```python
from build123d import *

# Parameters (mm, degrees)
SKETCH1_W           = 79
SKETCH1_H           = 46
SKETCH1_W_2         = 10
SKETCH1_H_2         = 7
SKETCH1_W_3         = 4
SKETCH1_H_3         = 5
BOSS_EXTRUDE1_DEPTH = 10


with BuildPart() as part:
    # Sketch1 → Boss-Extrude1 (new body)
    with BuildSketch(Plane.XY):
        with Locations((0, 20.611542264)):
            Rectangle(SKETCH1_W, SKETCH1_H)
        Polygon((-32.5, 38.111542264), (-36.5, 38.111542264), (-36.5, 33.111542264), (-32.5, 33.107370015), align=None, mode=Mode.SUBTRACT)
        with Locations((0, 5.111542264)):
            Rectangle(SKETCH1_W_2, SKETCH1_H_2, mode=Mode.SUBTRACT)
        with Locations((34.5, 35.607370015)):
            Rectangle(SKETCH1_W_3, SKETCH1_H_3, mode=Mode.SUBTRACT)
    extrude(amount=BOSS_EXTRUDE1_DEPTH)


solid = part.part
```
The listing builds one solid part. Answer for the finished solid, in the listing's coordinates (mm). A direction names the side the tool comes from. Give positions to 0.01 mm unless a question says otherwise; leave off trailing zeros. Order: outer loops, then holes, each group sorted by start corner. A loop starts at its lowest first (then second) coordinate and runs counter-clockwise, first axis right, second up. Notation, with made-up numbers: (38, 33) -> (54, 33) arc R33 ccw to (54, 67) -> close; hole circle Ø2 at (11, 17.5). An arc over 180 degrees is marked (long way). Answer as CSV lines item,"result". Start each with the question number.
Q1. A cutting plane is placed at C-C (z = 4.75). Determine the outline of the cut face in (x, y), then the cut area to 3 significant figures.
Q2. Which of the six approach directions +Z, -Z, +X, -X, +Y, -Y give full straight-line access (tool end or side, diameter ignored) to faces 1 (the flat face through (-1, 43.612, 5)), 2 (the flat face through (32.5, 36, 5))?
Q3. A cutting plane is placed at D-D (y = 36.5). Determine the outline of the cut face in (x, z).
Q4. A cutting plane is placed at A-A (x = 34.5). Determine the outline of the cut face in (y, z).
Q5. Determine the mould class of faces 3 (the flat face through (-39.5, 20, 5)), 4 (the flat face through (0, 1.612, 5)), 5 (the flat face through (39.5, 20, 5)), 6 (the flat face through (-1, 21, 10)) for opening direction X: pulls with the +X half, pulls with the -X half, needs draft (parallel to the pull), parting line crosses it, or undercut.
Q6. A cutting plane is placed at B-B (y = 2.5). Determine the outline of the cut face in (x, z).
Q7. Find the intervals of material crossed by L1, parallel to Y at x = 34.5, z = 3; L2, parallel to X at y = 7, z = 3; L3, parallel to Y at x = 4.5, z = 8.5, in increasing order.
Results found:
1,outline,"(-39.5, -2.39) -> (39.5, -2.39) -> (39.5, 43.61) -> (-39.5, 43.61) -> close; hole (-36.5, 33.11) -> (-32.5, 33.11) -> (-32.5, 38.11) -> (-36.5, 38.11) -> close; hole (-5, 1.61) -> (5, 1.61) -> (5, 8.61) -> (-5, 8.61) -> close; hole (32.5, 33.11) -> (36.5, 33.11) -> (36.5, 38.11) -> (32.5, 38.11) -> close"
1,area,"3,520 mm2"
2,face 1,"+Z, -Z, +X, -X, +Y"
2,face 2,"+Z, -Z"
3,outline,"(-39.5, 0) -> (-36.5, 0) -> (-36.5, 10) -> (-39.5, 10) -> close; (-32.5, 0) -> (32.5, 0) -> (32.5, 10) -> (-32.5, 10) -> close; (36.5, 0) -> (39.5, 0) -> (39.5, 10) -> (36.5, 10) -> close"
4,outline,"(-2.39, 0) -> (33.11, 0) -> (33.11, 10) -> (-2.39, 10) -> close; (38.11, 0) -> (43.61, 0) -> (43.61, 10) -> (38.11, 10) -> close"
5,face 3,"pulls with the -X half"
5,face 4,"undercut"
5,face 5,"pulls with the +X half"
5,face 6,"needs draft"
6,outline,"(-39.5, 0) -> (-5, 0) -> (-5, 10) -> (-39.5, 10) -> close; (5, 0) -> (39.5, 0) -> (39.5, 10) -> (5, 10) -> close"
7,L1,"-2.39 to 33.11, 38.11 to 43.61"
7,L2,"-39.5 to -5, 5 to 39.5"
7,L3,"-2.39 to 1.61, 8.61 to 43.61"
